```python
from build123d import *

# Parameters (mm, degrees)
BOSS_EXTRUDE1_DEPTH     = 1200
BOSS_EXTRUDE2_DEPTH     = 1200
CUT_EXTRUDE1_DEPTH      = 1230.636633319
CUT_EXTRUDE1_DEPTH_BACK = 1230.636633319
SKETCH2_W               = 1140
SKETCH2_H               = 120
CUT_EXTRUDE3_DEPTH      = 1230.636633319
SKETCH4_W               = 205
SKETCH4_H               = 50
CUT_EXTRUDE4_DEPTH      = 1230.636633319
CUT_EXTRUDE5_DEPTH      = 1230.636633319
CUT_EXTRUDE5_DEPTH_BACK = 1230.636633319
SKETCH5_R               = 3.05


with BuildPart() as part:
    # Sketch1 → Boss-Extrude1 (new body)
    with BuildSketch(Plane.XY):
        Polygon((122.5, 0), (152.5, 0), (222.5, 0), (222.5, -50), (-222.5, -50), (-222.5, 0), (-152.5, 0), (-122.5, 0), align=None)
    extrude(amount=BOSS_EXTRUDE1_DEPTH)

    # Sketch1_3 → Boss-Extrude2 (add)
    with BuildSketch(Plane.XY):
        Polygon((122.5, 0), (122.5, 120), (-122.5, 120), (-122.5, 0), (-152.5, 0), (-152.5, 150), (152.5, 150), (152.5, 0), align=None)
    extrude(amount=BOSS_EXTRUDE2_DEPTH)

    # Sketch2 → Cut-Extrude1 (cut, two sides: drawn at the far end of the back side and taken through both)
    with BuildSketch(Plane(origin=(0, 0, 0), x_dir=(0, 0, -1), z_dir=(1, 0, 0)).offset(-CUT_EXTRUDE1_DEPTH_BACK)):
        with Locations((-600, 60)):
            Rectangle(SKETCH2_W, SKETCH2_H)
    extrude(amount=CUT_EXTRUDE1_DEPTH + CUT_EXTRUDE1_DEPTH_BACK, mode=Mode.SUBTRACT)

    # Sketch3 → Cut-Extrude3 (cut, through all)
    with BuildSketch(Plane(origin=(0, 0, 0), x_dir=(1, 0, 0), z_dir=(0, 1, 0))):
        Polygon((-152.5, -30), (-222.5, -30), (-222.5, -1170), (-152.5, -1170), (152.5, -1170), (222.5, -1170), (222.5, -30), (152.5, -30), align=None)
    extrude(amount=-CUT_EXTRUDE3_DEPTH, mode=Mode.SUBTRACT)

    # Sketch4 → Cut-Extrude4 (cut, through all)
    with BuildSketch(Plane(origin=(0, 0, 0), x_dir=(1, 0, 0), z_dir=(0, 1, 0))):
        with Locations((0, -900)):
            Rectangle(SKETCH4_W, SKETCH4_H)
        with Locations((0, -300)):
            Rectangle(SKETCH4_W, SKETCH4_H)
    extrude(amount=CUT_EXTRUDE4_DEPTH, mode=Mode.SUBTRACT)

    # Sketch5 → Cut-Extrude5 (cut, two sides: drawn at the far end of the back side and taken through both)
    with BuildSketch(Plane(origin=(0, 0, 0), x_dir=(0, 0, -1), z_dir=(1, 0, 0)).offset(-CUT_EXTRUDE5_DEPTH_BACK)):
        with Locations(Location((-900, 135, 0), (0, 0, 180))):
            Circle(SKETCH5_R)
        with Locations(Location((-300, 135, 0), (0, 0, 180))):
            Circle(SKETCH5_R)
    extrude(amount=CUT_EXTRUDE5_DEPTH + CUT_EXTRUDE5_DEPTH_BACK, mode=Mode.SUBTRACT)


solid = part.part
```
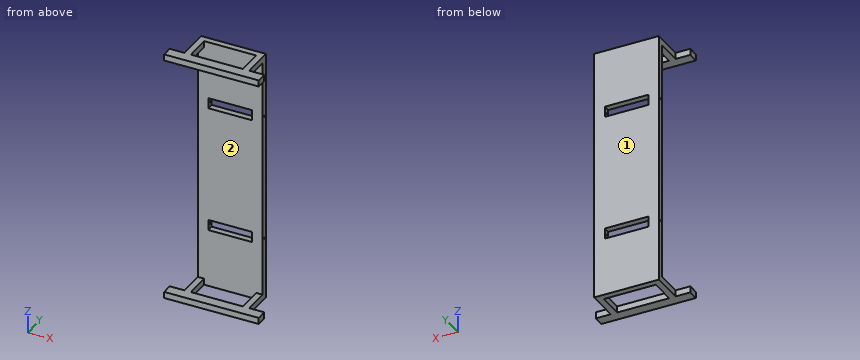
Can you work these out from the model? Positions are in its coordinate system, mm. Face numbers are marked on the shaded views. Give positions to 0.01 mm unless a question says otherwise; leave off trailing zeros. Loops run counter-clockwise (first coordinate to the right, second up) from the corner with the lowest first, then second, coordinate; pieces in that order, holes last. Notation, with made-up numbers: M 43.25,52.5 L 54.25,52.5 A11 cw 54.25,60.5 Z; hole C -37,33.25 d10. An arc over 180 degrees is marked long. Use CSV: the item, a comma, the result in double quotes. Start each with the question number.
1. For P1, Ø15, axis at x = 176.5, z = 1178.5, coming from the +Y side; P2, Ø9, axis at y = 140.5, z = 908, coming from the +X side; P3, Ø10, axis at x = 114, z = 813, coming from the -Y side, each with a flat end and sliding along its axis, tell me the tip position at first contact or that it passes through.
2. If we mould it in two halves opening along Z, with no side actions, what happens to the marked faces 1 and 2? For each: released by +Z, released by -Z, zero draft, split by the parting line, or undercut.
3. If I drill on L1, parallel to Z at x = 128, y = 135; L2, parallel to Z at x = -38, y = 120.5; L3, parallel to Y at x = -122, z = 300, over which ranges is the centre line in solid material (lowest first)?
4. Imagine slicing it at B-B, the plane y = 32.5. Write out the boundary of the cut face in (x, z).
5. Imagine slicing it at A-A, the plane x = -36. Write out the boundary of the cut face in (y, z), plus the area to 3 significant figures.
6. Imagine slicing it at C-C, the plane z = 151. Write out the boundary of the cut face in (x, y).
Response values:
1,P1,"y = 0"
1,P2,"x = 152.5"
1,P3,"y = 120"
2,face 1,"zero draft"
2,face 2,"undercut"
3,L1,"0 to 296.95, 303.05 to 896.95, 903.05 to 1200"
3,L2,"0 to 275, 325 to 875, 925 to 1200"
3,L3,"120 to 131.95, 138.05 to 150"
4,outline,"M -152.5,0 L -122.5,0 L -122.5,30 L -152.5,30 Z; M -152.5,1170 L -122.5,1170 L -122.5,1200 L -152.5,1200 Z; M 122.5,0 L 152.5,0 L 152.5,30 L 122.5,30 Z; M 122.5,1170 L 152.5,1170 L 152.5,1200 L 122.5,1200 Z"
5,outline,"M -50,0 L 0,0 L 0,30 L -50,30 Z; M -50,1170 L 0,1170 L 0,1200 L -50,1200 Z; M 120,0 L 150,0 L 150,275 L 120,275 Z; M 120,325 L 150,325 L 150,875 L 120,875 Z; M 120,925 L 150,925 L 150,1200 L 120,1200 Z"
5,area,"36,000 mm^2"
6,outline,"M -152.5,120 L 152.5,120 L 152.5,150 L -152.5,150 Z"
